Geometry: final body of the model. Coordinates: model frame, mm. A direction names the side the tool comes from. Give positions to 0.01 mm unless a question says otherwise; leave off trailing zeros. Loops run counter-clockwise (first coordinate to the right, second up) from the corner with the lowest first, then second, coordinate; pieces in that order, holes last. Notation, with made-up numbers: (-19.75, -3.75) -> (8.25, -3.75) arc R17 cw to (8.25, 24.25) -> close; hole circle Ø6 at (-24.75, -24.5). An arc over 180 degrees is marked (long way). Answer in a Markdown table with one row per item. Add a question column.
1) Line query: line 1 (X direction, y = 25.5, z = -12.5); line 2 (Y direction, x = 8, z = -4); line 3 (Y direction, x = 7.5, z = -12). Output: solid intervals per line, ascending. Write a range as from..to.
2) Access query for faces 1 (the flat face through (11.902, 71, 0)), 2 (the flat face through (-13.036, 71, 0)), 3 (the cylindrical face through (-1.73, -3.49, 7.81)). Directions: +Z, -Z, +X, -X, +Y, -Y. A direction counts if a zero-diameter tool reaches every point of the face in a straight line with its end or side. Return the directions, or none.
3) First-contact query: P1, Ø10, axis at x = 8.5, y = 18.5, coming from the +Z side; P2, Ø1.5, axis at y = 42.5, z = 7, coming from the -X side; P3, Ø3, axis at x = 5.5, z = -1.5, coming from the -Y side. Flat tips, straight axial feed; report the tip coordinate or a pass-through.
4) Section query A-A (x = 0). Return the cut outline in (y, z), plus the area to 3 significant figures.
5) Draft query along X for faces 4 (the flat face through (0, -3, 8.2)), 5 (the cylindrical face through (-2.981, 49.035, -13.423)), 6 (the flat face through (-11.902, 71, 0)). Return one class per face: +X half, -X half, draft (parallel to the pull), parting line (faces both ways), or undercut.
6) Section query B-B (y = 35.5). Return the cut outline in (x, z), plus the area to 3 significant figures.
Autodesk Inventor part; units mm, degrees
ref_plane "XZ Plane" through (0, 0, 0) normal (0, 1, 0) x (-1, 0, 0)
sketch "Sketch1" plane through (0, 0, 0) normal (0, 1, 0) x (-1, 0, 0)
  circle A0 centre (0, 0) radius 16
  dimension "d0" = 32
extrude "Extrusion1" add sketch "Sketch1" along normal blind 30.4
sketch "Sketch2" plane through (0, 30.4, 0) normal (0, 1, 0) x (1, 0, 0)
  circle A0 centre (0, 0) radius 13.75
  dimension "d3" = 27.5
extrude "Extrusion2" add sketch "Sketch2" along normal blind 37.8
sketch "Sketch3" plane through (0, 0, 0) normal (0, -1, 0) x (1, 0, 0)
  circle A0 centre (0, 0) radius 10
  dimension "d6" = 20
extrude "Extrusion3" add sketch "Sketch3" along normal blind 3
sketch "Sketch4" plane through (0, -3, 0) normal (0, -1, 0) x (1, 0, 0)
  circle A0 centre (0, 0) radius 8
  dimension "d9" = 16
extrude "Extrusion4" add sketch "Sketch4" along normal blind 1
sketch "Sketch5" plane through (0, -4, 0) normal (0, -1, 0) x (1, 0, 0)
  circle A0 centre (0, 0) radius 6
  dimension "d12" = 12
extrude "Extrusion5" add sketch "Sketch5" along normal blind 1
sketch "Sketch6" plane through (0, -5, 0) normal (0, -1, 0) x (1, 0, 0)
  circle A0 centre (0, 0) radius 3
  dimension "d15" = 6
extrude "Extrusion6" add sketch "Sketch6" along normal blind 14.3
sketch "Sketch7" plane through (0, 68.2, 0) normal (0, 1, 0) x (1, 0, 0)
  line L0 (-9.25, -6) -> (-10.75, -6)
  line L1 (-10.75, -6) -> (-10.75, 6)
  line L2 (-10.75, 6) -> (-9.25, 6)
  line L3 (-9.25, 6) -> (-9.25, -6)
  circle A0 centre (0, 0) radius 10
  line L4 (-9.25, -6) -> (-10.75, 6) construction
  line L5 (-10.75, -6) -> (-9.25, 6) construction
  point P0 (-10, 0)
  dimension "d18" = 12
  dimension "d19" = 1.5
extrude "Extrusion7" [suppressed]
sketch "Sketch8" plane through (-10.75, 68.2, -6) normal (-1, 0, 0) x (0, 0, 1)
  line L0 (1.5, 11.5) -> (10.5, 11.5)
  line L1 (10.5, 11.5) -> (10.5, 8.812)
  line L2 (10.5, 8.812) -> (1.5, 8.812)
  line L3 (1.5, 8.812) -> (1.5, 11.5)
  line L4 (0, 12.5) -> (12, 12.5)
  line L5 (0, 0) -> (0, 12.5)
  line L6 (12, 0) -> (12, 12.5)
  point P0 (6, -68.2)
  dimension "d22" = 1
  dimension "d23" = 1.5
  dimension "d24" = 1.5
extrude "Extrusion8" [suppressed]
sketch "Sketch9" plane through (0, 0, 0) normal (0, -1, 0) x (1, 0, 0)
  circle A0 centre (0, 0) radius 13.75
  line L0 (-9.4443, 9.9933) -> (9.4443, 9.9933)
  line L1 (9.4443, 9.9933) -> (9.4443, -9.9933)
  line L2 (9.4443, -9.9933) -> (-9.4443, -9.9933)
  line L3 (-9.4443, -9.9933) -> (-9.4443, 9.9933)
  line L4 (-9.4443, 9.9933) -> (9.4443, -9.9933) construction
  line L5 (9.4443, 9.9933) -> (-9.4443, -9.9933) construction
  circle A1 centre (9.4443, -9.9933) radius 0.5
  circle A2 centre (-9.4443, -9.9933) radius 0.5
  circle A3 centre (-9.4443, 9.9933) radius 0.5
  circle A4 centre (9.4443, 9.9933) radius 0.5
  dimension "d27" = 1
  dimension "d28" = 1
  dimension "d29" = 1
  dimension "d30" = 1
extrude "Extrusion9" cut sketch "Sketch9" against normal blind 1 contours A4 L1 A0 | A0 A4 | A1 A0 | A0 L1 A1 | L0 A4 A0 | L1 A4 L0 | L2 A1 L1 | A0 A1 L2 | A3 L0 A0 | A0 A3 | A3 L3 L0 | A2 A0 | A0 L2 A2 | L2 L3 A2 | L3 A3 A0 | A0 A2 L3
sketch "Sketch10" plane through (0, 0, 0) normal (0, -1, 0) x (1, 0, 0)
  circle A0 centre (0, 0) radius 16
  line L0 (0, 16) -> (0, 14.5)
  line L1 (0, 14.5) -> (-1, 14.5)
  line L2 (-1, 14.5) -> (-1, 16)
  line L3 (-1, 16) -> (0, 16)
  line L4 (0, 16) -> (0, 14.5)
  line L5 (0, 14.5) -> (1, 14.5)
  line L6 (1, 14.5) -> (1, 16)
  line L7 (1, 16) -> (0, 16)
  dimension "d33" = 1
  dimension "d34" = 1
  dimension "d35" = 1.5
extrude "Extrusion10" cut sketch "Sketch10" against normal blind 1 contours L6 L5 L0 A0 | A0 L7 L6 | L2 L3 A0 | A0 L0 L1 L2
mirror "Mirror1" about plane through (0, 0, 0) normal (0, 0, 1) of "Extrusion10"
sketch "Sketch11" plane through (0, 0, 0) normal (0, -1, 0) x (1, 0, 0)
  arc A0 (1, -15.9687) -> (1, 15.9687) centre (0, 0) ccw
  line L0 (16, 0) -> (14.5, 0)
  line L1 (14.5, 0) -> (14.5, 1)
  line L2 (14.5, 1) -> (16, 1)
  line L3 (16, 1) -> (16, 0)
  line L4 (16, 0) -> (14.5, 0)
  line L5 (14.5, 0) -> (14.5, -1)
  line L6 (14.5, -1) -> (16, -1)
  line L7 (16, -1) -> (16, 0)
  dimension "d38" = 1
  dimension "d39" = 1
  dimension "d40" = 1.5
extrude "Extrusion11" cut sketch "Sketch11" against normal blind 1
mirror "Mirror2" about plane through (0, 0, 0) normal (1, 0, 0) of "Extrusion11"
sketch "Sketch12" plane through (0, 68.2, 0) normal (0, 1, 0) x (1, 0, 0)
  line L0 (-13.0359, 2.9472) -> (-13.0359, -2.9472)
  line L1 (-13.0359, -2.9472) -> (-11.9023, -2.9472)
  line L2 (-11.9023, -2.9472) -> (-11.9023, 2.9472)
  line L3 (-11.9023, 2.9472) -> (-13.0359, 2.9472)
  line L4 (-13.0359, 2.9472) -> (-11.9023, -2.9472) construction
  line L5 (-13.0359, -2.9472) -> (-11.9023, 2.9472) construction
  point P0 (0, 0)
  point P1 (-12.4691, 0)
extrude "Extrusion12" add sketch "Sketch12" along normal blind 6
ref_plane "Work Plane1" through (0, 30.4, 13.75) normal (0, 0, 1) x (1, 0, 0)
ref_plane "Work Plane3" through (0, 30.4, 0) normal (0, 0, 1) x (1, 0, 0)
ref_plane "Work Plane2" through (0, 30.4, -13.75) normal (0, 0, 1) x (1, 0, 0)
ref_plane "Work Plane4" through (-13.75, 30.4, 0) normal (1, 0, 0) x (0, 1, 0)
ref_plane "Work Plane6" through (0, 30.4, 0) normal (1, 0, 0) x (0, 1, 0)
ref_plane "Work Plane5" through (13.75, 30.4, 0) normal (1, 0, 0) x (0, 1, 0)
mirror "Mirror3" about plane through (0, 30.4, 0) normal (1, 0, 0) of "Extrusion12"
properties part number "Drive Motor"
Evaluation:
| question | item | result |
|---|---|---|
| 1 | line 1 | -9.99..9.99 |
| 1 | line 2 | -3..68.2 |
| 1 | line 3 | 0..30.4 |
| 2 | face 1 | +Z, -Z, +Y |
| 2 | face 2 | +Z, -Z, -X, +Y |
| 2 | face 3 | -Y |
| 3 | P1 | z = 15.61 |
| 3 | P2 | x = -12.25 |
| 3 | P3 | y = -5 |
| 4 | outline | (-19.3, -3) -> (-5, -3) -> (-5, -6) -> (-4, -6) -> (-4, -8) -> (-3, -8) -> (-3, -10) -> (0, -10) -> (0, -14.5) -> (1, -14.5) -> (1, -16) -> (30.4, -16) -> (30.4, -13.75) -> (68.2, -13.75) -> (68.2, 13.75) -> (30.4, 13.75) -> (30.4, 16) -> (1, 16) -> (1, 14.5) -> (0, 14.5) -> (0, 10) -> (-3, 10) -> (-3, 8) -> (-4, 8) -> (-4, 6) -> (-5, 6) -> (-5, 3) -> (-19.3, 3) -> close |
| 4 | area | 2,180 mm² |
| 5 | face 4 | draft |
| 5 | face 5 | parting line |
| 5 | face 6 | undercut |
| 6 | outline | circle Ø27.5 at (0, 0) |
| 6 | area | 594 mm² |
